from build123d import *

# Parameters (mm, degrees)
SKETCH1_R           = 1.5
BOSS_EXTRUDE1_DEPTH = 2
CUT_EXTRUDE1_DEPTH  = 197.459257863
CHAMFER1_SIZE       = 2
BOSS_EXTRUDE2_DEPTH = 2
CUT_EXTRUDE2_DEPTH  = 197.398014273
SKETCH5_R           = 1.85
CUT_EXTRUDE3_DEPTH  = 197.398014273


with BuildPart() as part:
    # Sketch1 → Boss-Extrude1 (new body)
    with BuildSketch(Plane.XY):
        with BuildLine():
            Line((102.318351238, 102.318351238), (113.419927702, 113.419927702))
            ThreePointArc((113.419927702, 113.419927702), (160.4, 0), (113.419927702, -113.419927702))
            Line((113.419927702, -113.419927702), (102.318351238, -102.318351238))
            ThreePointArc((102.318351238, -102.318351238), (144.7, 0), (102.318351238, 102.318351238))
        make_face()
        with Locations((121.321245866, 98.702154493)):
            Circle(SKETCH1_R, mode=Mode.SUBTRACT)
        with Locations((143.451847555, 62.309930452)):
            Circle(SKETCH1_R, mode=Mode.SUBTRACT)
        with Locations((154.94328196, 21.296463919)):
            Circle(SKETCH1_R, mode=Mode.SUBTRACT)
        with Locations((154.94328196, -21.296463919)):
            Circle(SKETCH1_R, mode=Mode.SUBTRACT)
        with Locations((143.451847555, -62.309930452)):
            Circle(SKETCH1_R, mode=Mode.SUBTRACT)
        with Locations((121.321245866, -98.702154493)):
            Circle(SKETCH1_R, mode=Mode.SUBTRACT)
        with Locations(Location((127.774091267, 90.192802379, 0), (0, 0, 180))):
            Circle(SKETCH1_R, mode=Mode.SUBTRACT)
        with Locations(Location((147.369608219, 52.375171344, 0), (0, 0, 180))):
            Circle(SKETCH1_R, mode=Mode.SUBTRACT)
        with Locations(Location((153.128751314, 31.820520441, 0), (0, 0, 180))):
            Circle(SKETCH1_R, mode=Mode.SUBTRACT)
        with Locations(Location((156.035395501, 10.67311345, 0), (0, 0, 180))):
            Circle(SKETCH1_R, mode=Mode.SUBTRACT)
        with Locations(Location((127.774091267, -90.192802379, 0), (0, 0, 180))):
            Circle(SKETCH1_R, mode=Mode.SUBTRACT)
        with Locations(Location((147.369608219, -52.375171344, 0), (0, 0, 180))):
            Circle(SKETCH1_R, mode=Mode.SUBTRACT)
        with Locations(Location((153.128751314, -31.820520441, 0), (0, 0, 180))):
            Circle(SKETCH1_R, mode=Mode.SUBTRACT)
        with Locations(Location((156.035395501, -10.67311345, 0), (0, 0, 180))):
            Circle(SKETCH1_R, mode=Mode.SUBTRACT)
        with Locations((138.865248158, 71.954171901)):
            Circle(SKETCH1_R, mode=Mode.SUBTRACT)
        with Locations((114.302744813, 106.751311599)):
            Circle(SKETCH1_R, mode=Mode.SUBTRACT)
        with Locations((138.865248158, -71.954171901)):
            Circle(SKETCH1_R, mode=Mode.SUBTRACT)
        with Locations((114.302744813, -106.751311599)):
            Circle(SKETCH1_R, mode=Mode.SUBTRACT)
    extrude(amount=BOSS_EXTRUDE1_DEPTH)

    # Sketch2 → Cut-Extrude1 (cut, through all)
    with BuildSketch(Plane.XY.offset(2)):
        Polygon((117.10590357, 116.893771535), (92.696291985, 92.484159951), (81.614099529, 103.566352407), (106.023711114, 127.975963992), align=None)
        Polygon((94.953094668, -94.740962634), (127.588403443, -127.376271408), (106.110382849, -148.854292002), (73.475074075, -116.218983227), align=None)
    extrude(amount=-CUT_EXTRUDE1_DEPTH, mode=Mode.SUBTRACT)

    # Chamfer1
    chamfer1_edges = [part.edges().sort_by_distance(p)[0] for p in [
        (119.821245866, 98.702154493, 2),
        (141.951847555, 62.309930452, 2),
        (153.44328196, 21.296463919, 2),
        (153.44328196, -21.296463919, 2),
        (141.951847555, -62.309930452, 2),
        (119.821245866, -98.702154493, 2),
        (129.274091267, 90.192802379, 2),
        (148.869608219, 52.375171344, 2),
        (154.628751314, 31.820520441, 2),
        (157.535395501, 10.67311345, 2),
        (129.274091267, -90.192802379, 2),
        (148.869608219, -52.375171344, 2),
        (154.628751314, -31.820520441, 2),
        (157.535395501, -10.67311345, 2),
        (112.802744813, 106.751311599, 2),
        (137.365248158, 71.954171901, 2),
        (137.365248158, -71.954171901, 2),
        (112.802744813, -106.751311599, 2),
    ]]
    chamfer(chamfer1_edges, length=CHAMFER1_SIZE - 0.0001)  # a hair under: the kernel refuses the full size

    # Sketch3 → Boss-Extrude2 (add)
    with BuildSketch(Plane(origin=(0, 0, 0), x_dir=(-1, 0, 0), z_dir=(0, 0, -1))):
        with BuildLine():
            ThreePointArc((-133.156583772, -89.428654235), (-140.426335781, -106.48865188), (-122.037613507, -104.091214277))
            ThreePointArc((-122.037613507, -104.091214277), (-127.807539871, -96.919516879), (-133.156583772, -89.428654235))
        make_face()
        with BuildLine():
            ThreePointArc((-122.037613507, 104.091214277), (-140.426335781, 106.48865188), (-133.156583772, 89.428654235))
            ThreePointArc((-133.156583772, 89.428654235), (-127.807539871, 96.919516879), (-122.037613507, 104.091214277))
        make_face()
    extrude(amount=-BOSS_EXTRUDE2_DEPTH)

    # Sketch4 → Cut-Extrude2 (cut, through all)
    with BuildSketch(Plane(origin=(0, 0, 0), x_dir=(-1, 0, 0), z_dir=(0, 0, -1))):
        with BuildLine():
            ThreePointArc((-122.037613507, -104.091214277), (-135.141839583, -102.481291915), (-133.156583772, -89.428654235))
            ThreePointArc((-133.156583772, -89.428654235), (-147.070909653, -111.527391302), (-122.037613507, -104.091214277))
        make_face()
        with BuildLine():
            ThreePointArc((-133.156583772, 89.428654235), (-135.141839583, 102.481291915), (-122.037613507, 104.091214277))
            ThreePointArc((-122.037613507, 104.091214277), (-145.081010417, 110.018403078), (-133.156583772, 89.428654235))
        make_face()
    extrude(amount=-CUT_EXTRUDE2_DEPTH, mode=Mode.SUBTRACT)

    # Sketch5 → Cut-Extrude3 (cut, through all)
    with BuildSketch(Plane(origin=(0, 0, 0), x_dir=(-1, 0, 0), z_dir=(0, 0, -1))):
        with Locations((-131.954619137, -100.064346357)):
            Circle(SKETCH5_R)
        with Locations((-131.954619137, 100.064346357)):
            Circle(SKETCH5_R)
    extrude(amount=-CUT_EXTRUDE3_DEPTH, mode=Mode.SUBTRACT)


solid = part.part
CAD build for the part. Positions are in the model's coordinates, mm. A direction names the side the tool comes from. Coordinates: 2 decimals unless noted, no trailing zeros. One line per item, written item: value.
1. Pull direction Y, two halves, no side cores. Call faces 1 (the face through (130.19, 100.62, 0.99)), 2 (the face through (108.05, 107.84, 1.01)), 3 (the face through (107.9, -107.69, 1.01)): pulls with the +Y half, pulls with the -Y half, needs draft (parallel to the pull), parting line crosses it, or undercut.
Answers:
face 1: undercut
face 2: pulls with the +Y half
face 3: pulls with the -Y half
2. Drill centre lines: line 1 (Y direction, x = 133.5, z = 0.25); line 2 (Y direction, x = 145, z = 1.8); line 3 (Y direction, x = 148.5, z = 0.65). Where is each one in solid material? Low to high. Write a range as [from, to].
Answers:
line 1: y = [-104.15, -101.08], [-99.05, -89.69], [-88.92, -55.82], [55.82, 88.92], [89.69, 99.05], [101.08, 104.15]
line 2: y = [-68.58, -65.22], [-59.4, -54.67], [-50.08, 50.08], [54.67, 59.4], [65.22, 68.58]
line 3: y = [-60.63, -54.2], [-50.55, 50.55], [54.2, 60.63]
3. Flat gauge pins, fed straight in: P1, Ø1.8, axis at x = 143.45, y = -62.31, coming from the +Z side; P2, Ø5, axis at x = 154.94, y = 21.3, coming from the +Z side; P3, Ø3.5, axis at x = 121.32, y = -98.7, coming from the -Z side; P4, Ø3.5, axis at x = 127.77, y = -90.19, coming from the +Z side. Where does each tip first touch, or does it go through?
Answers:
P1: passes through
P2: stops at z = 1
P3: stops at z = 0
P4: stops at z = 0.26
4. Slice it at A-A on z = 0.45. Give the number of separate pieces and of enclosed holes in the cut face, and give its area (3 significant figures).
Answers:
separate pieces: 1
enclosed holes: 20
area: 3,790 mm^2
5. Which spindle directions (+Z, -Z, +X, -X, +Y, -Y) get a long thin tool onto all of the face, cutting with end or side? Do faces 4 (the face through (117.93, -108.72, 0.99)), 5 (the face through (130.246, -100.773, 0.986)), 6 (the face through (117.81, 108.85, 0.99)). Say none if no direction does.
Answers:
face 4: +Z, -Z, -Y
face 5: +Z, -Z
face 6: +Z, -Z, +Y
